Check sheet for the modelled part. Datum: model origin and axes. Units: mm. Face numbers are marked on the shaded views. A direction names the side the tool comes from. Round coordinates to 2 decimals unless told otherwise and drop trailing zeros. Order: outer loops, then holes, each group sorted by start corner. A loop starts at its lowest first (then second) coordinate and runs counter-clockwise, first axis right, second up. Notation, with made-up numbers: (6, 32) -> (52, 32) arc R9 cw to (52, 43) -> close; hole circle Ø8 at (-36, 72.25). An arc over 180 degrees is marked (long way). Answer in a Markdown table with one row per item.
```python
from build123d import *

# Parameters (mm, degrees)
F0_W     = 76.2
F0_H     = 63.5
F1_DEPTH = 6.35
F2_T     = -1.27
F3_R     = 3.175
F3_R_2   = 1.651
F4_DEPTH = 11.43
F5_W     = 48.26
F5_H     = 3.81
F5_W_2   = 39.37
F6_DEPTH = 1.27


# Not quite as in the source:
# - a feature names something its author has since deleted; it is built from what else it names


with BuildPart() as f1:
    # F0 (on Front) → F1 (new body)
    with BuildSketch(Plane.XZ):
        with Locations((38.1, 31.75)):
            Rectangle(F0_W, F0_H)
    extrude(amount=F1_DEPTH)

    # F2
    f2_openings = [f1.faces().sort_by_distance(p)[0] for p in [
        (38.1, -6.35, 31.75),
    ]]
    offset(amount=F2_T, openings=f2_openings)

    # F3 (on face) → F4 (join)
    with BuildSketch(Plane.XZ.offset(1.27)):
        with Locations((16.51, 55.3212)):
            Circle(F3_R)
        with Locations((16.51, 55.3212)):
            Circle(F3_R_2, mode=Mode.SUBTRACT)
        with Locations((68.58, 50.2412)):
            Circle(F3_R)
        with Locations((68.58, 50.2412)):
            Circle(F3_R_2, mode=Mode.SUBTRACT)
        with Locations((68.58, 22.3012)):
            Circle(F3_R)
        with Locations((68.58, 22.3012)):
            Circle(F3_R_2, mode=Mode.SUBTRACT)
        with Locations((17.78, 7.0612)):
            Circle(F3_R)
        with Locations((17.78, 7.0612)):
            Circle(F3_R_2, mode=Mode.SUBTRACT)
    extrude(amount=F4_DEPTH)

    # F5 (on face) → F6 (cut)
    with BuildSketch(Plane(origin=(0, 0, 0), x_dir=(-1, 0, 0), z_dir=(0, 1, 0))):
        with Locations((-45.212, 6.985)):
            Rectangle(F5_W, F5_H)
        with Locations((-49.657, 55.245)):
            Rectangle(F5_W_2, F5_H)
    extrude(amount=-F6_DEPTH, mode=Mode.SUBTRACT)


solid = f1.part
```
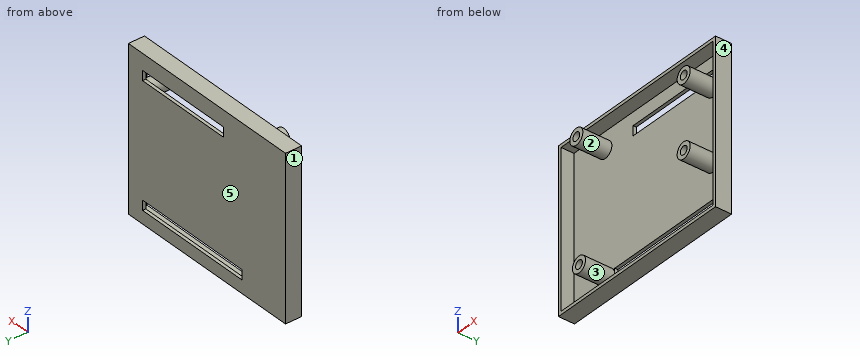
(1) Tool access check on the marked faces 1 and 2. Record the directions out of +Z, -Z, +X, -X, +Y, -Y that give a thin tool (end or side, any length) a straight path to the whole face; none if there is none.
Solutions:
| item | result |
|---|---|
| face 1 | +Z, -Z, -X, +Y, -Y |
| face 2 | -Y |
(2) Scan lines: probe 1 along Z at (x, y) = (68.58, -7.75); probe 2 along X at (y, z) = (-6, 55.5); probe 3 along X at (y, z) = (-4.5, 28.5). Record each from-to range of solid material in increasing order. Write a range as from..to.
Solutions:
| item | result |
|---|---|
| probe 1 | 19.13..20.65, 23.95..25.48, 47.07..48.59, 51.89..53.42 |
| probe 2 | 0..1.27, 13.34..14.87, 18.15..19.68, 74.93..76.2 |
| probe 3 | 0..1.27, 74.93..76.2 |
(3) Section check C-C on x = 11.5. Record the boundary of the cut face in (y, z).
Solutions:
| item | result |
|---|---|
| outline | (-6.35, 0) -> (0, 0) -> (0, 63.5) -> (-6.35, 63.5) -> (-6.35, 62.23) -> (-1.27, 62.23) -> (-1.27, 1.27) -> (-6.35, 1.27) -> close |
(4) Draft check along X on the marked faces 3, 4 and 5. Enter one of: pulls with the +X half, pulls with the -X half, needs draft (parallel to the pull), parting line crosses it, or undercut.
Solutions:
| item | result |
|---|---|
| face 3 | undercut |
| face 4 | pulls with the +X half |
| face 5 | needs draft |
(5) Depth check by flat-ended pin: pin 1 Ø6 at (x, z) = (29.5, 42.5) entering from -Y. Enter the tip coordinate at first touch or a pass-through.
Solutions:
| item | result |
|---|---|
| pin 1 | y = -1.27 |
(6) Section check A-A on y = -10. Record the boundary of the cut face in (x, z) (3 decimals), plus the area to 3 significant figures.
Solutions:
| item | result |
|---|---|
| outline | circle Ø6.35 at (16.51, 55.321); circle Ø6.35 at (17.78, 7.061); circle Ø6.35 at (68.58, 22.301); circle Ø6.35 at (68.58, 50.241); hole circle Ø3.302 at (16.51, 55.321); hole circle Ø3.302 at (17.78, 7.061); hole circle Ø3.302 at (68.58, 22.301); hole circle Ø3.302 at (68.58, 50.241) |
| area | 92.4 mm^2 |
(7) Section check B-B on y = -3. Give the number of separate pieces and of enclosed holes in the cut face, plus the area to 3 significant figures.
Solutions:
| item | result |
|---|---|
| separate pieces | 5 |
| enclosed holes | 5 |
| area | 441 mm^2 |
